```python
from build123d import *

# Parameters (mm, degrees)
F0_R     = 2.475
F1_DEPTH = 6
F2_R     = 2.975
F3_DEPTH = 12
F4_R     = 2.35
F5_DEPTH = 6
F6_R     = 0.1


with BuildPart() as f1:
    # F0 (on Top) → F1 (new body)
    with BuildSketch(Plane.XY):
        Circle(F0_R)
    extrude(amount=F1_DEPTH)

    # F2 (on face) → F3 (join)
    with BuildSketch(Plane.XY.offset(6)):
        Circle(F2_R)
    extrude(amount=F3_DEPTH)

    # F4 (on face) → F5 (cut)
    with BuildSketch(Plane.XY.offset(18)):
        Circle(F4_R)
    extrude(amount=-F5_DEPTH, mode=Mode.SUBTRACT)

    # F6
    f6_edges = [f1.edges().sort_by_distance(p)[0] for p in [
        (-2.475, 0, 0),
        (-2.975, 0, 18),
        (-2.35, 0, 18),
        (-2.975, 0, 6),
        (-2.475, 0, 6),
    ]]
    fillet(f6_edges, radius=F6_R)


solid = f1.part
```
CAD build for the part. Positions are in the model's coordinates, mm. Give positions to 0.01 mm unless a question says otherwise; leave off trailing zeros. Loops run counter-clockwise (first coordinate to the right, second up) from the corner with the lowest first, then second, coordinate; pieces in that order, holes last. Notation, with made-up numbers: (-12.5, 30.25) -> (6.5, 30.25) arc R26 ccw to (6.5, 58.25) -> close; hole circle Ø1 at (-16, -15.75). An arc over 180 degrees is marked (long way). Use a Markdown table: item, result.
1. Slice it at A-A (y = 0). List the corners of the cut face in (x, z) (3 decimals).
Check result:
| item | result |
|---|---|
| outline | (-2.975, 6.1) arc R0.1 ccw to (-2.875, 6) -> (-2.575, 6) arc R0.1 cw to (-2.475, 5.9) -> (-2.475, 0.1) arc R0.1 ccw to (-2.375, 0) -> (2.375, 0) arc R0.1 ccw to (2.475, 0.1) -> (2.475, 5.9) arc R0.1 cw to (2.575, 6) -> (2.875, 6) arc R0.1 ccw to (2.975, 6.1) -> (2.975, 17.9) arc R0.1 ccw to (2.875, 18) -> (2.45, 18) arc R0.1 ccw to (2.35, 17.9) -> (2.35, 12) -> (-2.35, 12) -> (-2.35, 17.9) arc R0.1 ccw to (-2.45, 18) -> (-2.875, 18) arc R0.1 ccw to (-2.975, 17.9) -> close |
2. Wall check: L1, parallel to Y at x = 0, z = 16.75 (3 decimals); L2, parallel to Z at x = -0.3, y = -2.65; L3, parallel to Z at x = 1.4, y = -0.1. Give the ranges that are in metal, low to high. Write a range as [from, to].
Check result:
| item | result |
|---|---|
| L1 | y = [-2.975, -2.35], [2.35, 2.975] |
| L2 | z = [6, 18] |
| L3 | z = [0, 12] |
3. Mould opens along X. For faces 1 (the cylindrical face through (2.36, 0.74, 2.96)), 2 (the flat face through (0, 0, 12)), 3 (the cylindrical face through (-0.509, -2.294, 14.991)), 4 (the flat face through (0, 0, 0)) say: pulls with the +X half, pulls with the -X half, needs draft (parallel to the pull), parting line crosses it, or undercut.
Check result:
| item | result |
|---|---|
| face 1 | parting line crosses it |
| face 2 | undercut |
| face 3 | undercut |
| face 4 | needs draft |
4. Flat gauge pins, fed straight in: pin 1 (1 mm diameter, centred on x = -1, y = 1, fed in from +Z); pin 2 (2 mm diameter, centred on y = -2, z = 10.5, fed in from +X). Where does each tip first touch, or does it go through?
Check result:
| item | result |
|---|---|
| pin 1 | stops at z = 12 |
| pin 2 | stops at x = 2.8 |
5. Slice it at D-D (z = 14.25). List the corners of the cut face in (x, y) (3 decimals), plus the area to 3 significant figures.
Check result:
| item | result |
|---|---|
| outline | circle Ø5.95 at (0, 0); hole circle Ø4.7 at (0, 0) |
| area | 10.5 mm^2 |
6. Slice it at C-C (z = 4). List the corners of the cut face in (x, y) (3 decimals), plus the area to 3 significant figures.
Check result:
| item | result |
|---|---|
| outline | circle Ø4.95 at (0, 0) |
| area | 19.2 mm^2 |
